```python
from build123d import *

# Parameters (mm, degrees)
EXTRUDE_1_DEPTH          = 20
CUT_EXTRUDE_2_DEPTH      = 60.371710435
CUT_EXTRUDE_2_DEPTH_BACK = 60.371710435
SKETCH_3_R               = 1.65
SKETCH_4_W               = 13
SKETCH_4_H               = 20
EXTRUDE_2_DEPTH          = 5
CUT_EXTRUDE_3_DEPTH      = 65.915329468
CUT_EXTRUDE_3_DEPTH_BACK = 65.915329468
SKETCH_5_R               = 1.65
CUT_EXTRUDE_6_DEPTH      = 64.356136246
CUT_EXTRUDE_6_DEPTH_BACK = 64.356136246
SKETCH_2_R               = 1.5


with BuildPart() as part:
    # 草图1 → 凸台-拉伸1 (new body)
    with BuildSketch(Plane.XY):
        Polygon((0, 50), (0, 0), (30, 0), (30, 5), (7, 5), (5, 7), (5, 50), align=None)
    extrude(amount=EXTRUDE_1_DEPTH)

    # 草图3 → 切除-拉伸2 (cut, two sides: drawn at the far end of the back side and taken through both)
    with BuildSketch(Plane(origin=(5, 0, 0), x_dir=(0, 0, -1), z_dir=(1, 0, 0)).offset(-CUT_EXTRUDE_2_DEPTH_BACK)):
        with Locations(Location((-4, 46, 0), (0, 0, 90))):
            Circle(SKETCH_3_R)
        with Locations(Location((-16, 46, 0), (0, 0, 90))):
            Circle(SKETCH_3_R)
        with Locations(Location((-4, 32, 0), (0, 0, 90))):
            Circle(SKETCH_3_R)
        with Locations(Location((-16, 32, 0), (0, 0, 90))):
            Circle(SKETCH_3_R)
        with Locations(Location((-16, 18, 0), (0, 0, 90))):
            Circle(SKETCH_3_R)
        with Locations(Location((-4, 18, 0), (0, 0, 90))):
            Circle(SKETCH_3_R)
    extrude(amount=CUT_EXTRUDE_2_DEPTH + CUT_EXTRUDE_2_DEPTH_BACK, mode=Mode.SUBTRACT)

    # 草图4 → 凸台-拉伸2 (add)
    with BuildSketch(Plane.ZY):
        with Locations((26.5, 40)):
            Rectangle(SKETCH_4_W, SKETCH_4_H)
        with Locations((-6.5, 40)):
            Rectangle(SKETCH_4_W, SKETCH_4_H)
    extrude(amount=-EXTRUDE_2_DEPTH)

    # 草图5 → 切除-拉伸3 (cut, two sides: drawn at the far end of the back side and taken through both)
    with BuildSketch(Plane(origin=(5, 0, 0), x_dir=(0, 0, -1), z_dir=(1, 0, 0)).offset(-CUT_EXTRUDE_3_DEPTH_BACK)):
        with Locations(Location((-28, 46, 0), (0, 0, 90))):
            Circle(SKETCH_5_R)
        with Locations(Location((-28, 36, 0), (0, 0, 90))):
            Circle(SKETCH_5_R)
        with Locations(Location((8, 46, 0), (0, 0, 90))):
            Circle(SKETCH_5_R)
        with Locations(Location((8, 36, 0), (0, 0, 90))):
            Circle(SKETCH_5_R)
    extrude(amount=CUT_EXTRUDE_3_DEPTH + CUT_EXTRUDE_3_DEPTH_BACK, mode=Mode.SUBTRACT)

    # 草图2 → 切除-拉伸6 (cut, two sides: drawn at the far end of the back side and taken through both)
    with BuildSketch(Plane(origin=(0, 5, 0), x_dir=(1, 0, 0), z_dir=(0, 1, 0)).offset(-CUT_EXTRUDE_6_DEPTH_BACK)):
        with Locations(Location((9.48, -17.5, 0), (0, 0, 180))):
            Circle(SKETCH_2_R)
        with Locations(Location((19.48, -17.5, 0), (0, 0, 180))):
            Circle(SKETCH_2_R)
        with Locations(Location((19.48, -2.5, 0), (0, 0, 180))):
            Circle(SKETCH_2_R)
        with Locations(Location((9.48, -2.5, 0), (0, 0, 180))):
            Circle(SKETCH_2_R)
    extrude(amount=CUT_EXTRUDE_6_DEPTH + CUT_EXTRUDE_6_DEPTH_BACK, mode=Mode.SUBTRACT)


solid = part.part
```
CAD build for the part. Positions are in the model's coordinates, mm. A direction names the side the tool comes from. Round coordinates to 2 decimals unless told otherwise and drop trailing zeros. Order: outer loops, then holes, each group sorted by start corner. A loop starts at its lowest first (then second) coordinate and runs counter-clockwise, first axis right, second up.
Q1. Slice it at D-D (z = 10.5). Write the cut outline in (x, y), and give its area (3 significant figures).
Q2. Slice it at C-C (z = 5). Write the cut outline in (x, y), and give its area (3 significant figures).
Q3. Drop flat-ended pins along their axis: pin 1 (10 mm diameter, centred on x = 5, y = 9.5, fed in from -Z); pin 2 (2.5 mm diameter, centred on x = 3.5, z = -9.5, fed in from -Y); pin 3 (1.5 mm diameter, centred on y = 9, z = 6, fed in from +X). Give the stop position or say it passes through.
Q4. Two-plate mould, pull along Z, no slides. Class faces 1 (the flat face through (4, 11, 20)), 2 (the flat face through (19, 5, 10)), 3 (the cylindrical face through (2.47, 16.69, 3)), 4 (the cylindrical face through (2.47, 34.35, -7.93)): pulls with the +Z half, pulls with the -Z half, needs draft (parallel to the pull), parting line crosses it, or undercut.
Q5. Wall check: L1, parallel to Z at x = 3.75, y = 32; L2, parallel to X at y = 4.05, z = 17.5; L3, parallel to Y at x = 2.6, z = 28. Give the ranges that are in metal, low to high.
Q6. Slice it at B-B (y = 18). Write the cut outline in (x, z).
Q7. Which spindle directions (+Z, -Z, +X, -X, +Y, -Y) get a long thin tool onto all of the face, cutting with end or side? Do faces 5 (the flat face through (2, 30, 26)), 6 (the flat face through (2, 30, -7)), 7 (the cylindrical face through (2.47, 30.35, 16.07)). Say none if no direction does.
Q8. Slice it at A-A (z = -8). Write the cut outline in (x, y).
Results below:
1. outline: (0, 0) - (30, 0) - (30, 5) - (7, 5) - (5, 7) - (5, 50) - (0, 50) - close
1. area: 377 mm2
2. outline: (0, 0) - (30, 0) - (30, 5) - (7, 5) - (5, 7) - (5, 16.69) - (0, 16.69) - close; (0, 19.31) - (5, 19.31) - (5, 30.69) - (0, 30.69) - close; (0, 33.31) - (5, 33.31) - (5, 44.69) - (0, 44.69) - close; (0, 47.31) - (5, 47.31) - (5, 50) - (0, 50) - close
2. area: 338 mm2
3. pin 1: stops at z = 0
3. pin 2: stops at y = 30
3. pin 3: stops at x = 5
4. face 1: pulls with the +Z half
4. face 2: needs draft
4. face 3: undercut
4. face 4: undercut
5. L1: z = -13 to 2.35, 5.65 to 14.35, 17.65 to 33
5. L2: x = 0 to 7.98, 10.98 to 17.98, 20.98 to 30
5. L3: y = 30 to 34.35, 37.65 to 44.35, 47.65 to 50
6. outline: (0, 0) - (5, 0) - (5, 2.35) - (0, 2.35) - close; (0, 5.65) - (5, 5.65) - (5, 14.35) - (0, 14.35) - close; (0, 17.65) - (5, 17.65) - (5, 20) - (0, 20) - close
7. face 5: +Z, +X, -X, -Y
7. face 6: -Z, +X, -X, -Y
7. face 7: +X, -X
8. outline: (0, 30) - (5, 30) - (5, 34.35) - (0, 34.35) - close; (0, 37.65) - (5, 37.65) - (5, 44.35) - (0, 44.35) - close; (0, 47.65) - (5, 47.65) - (5, 50) - (0, 50) - close
